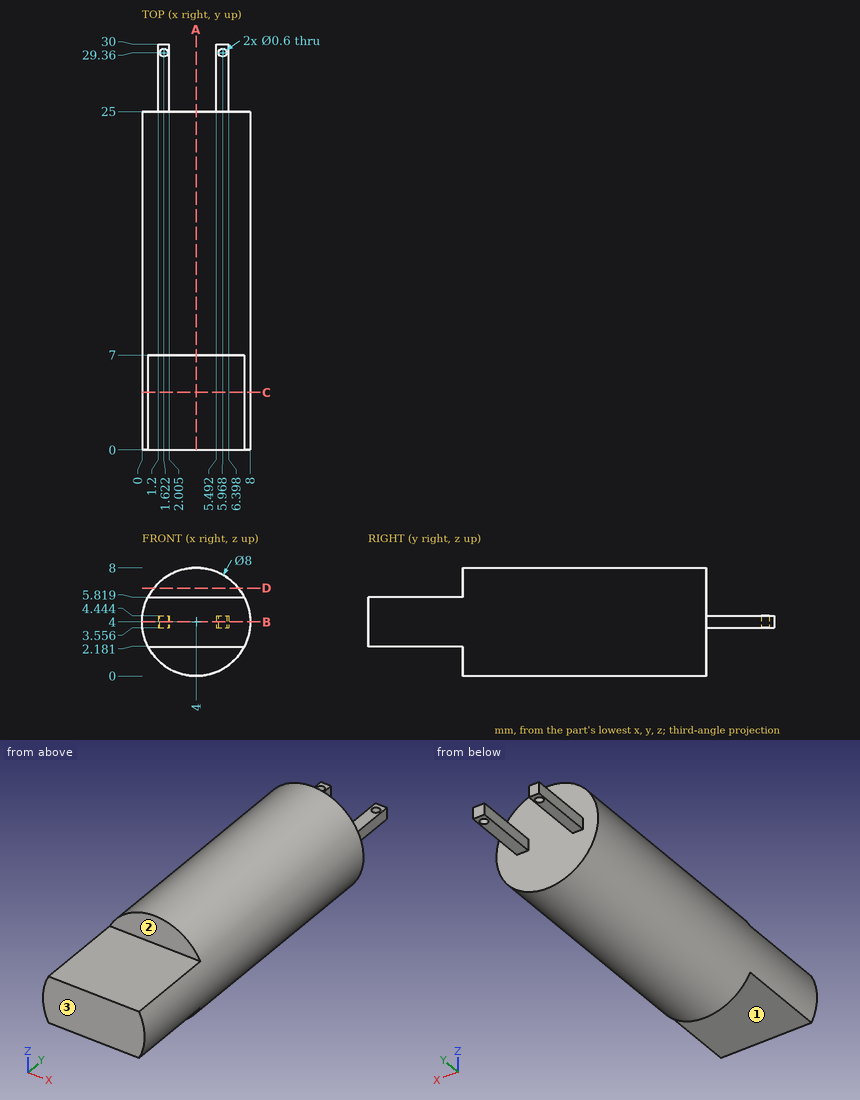
For this review, use the dimensioned drawing (mm, ordinates from the lowest corner) and the shaded views. A direction names the side the tool comes from. Give positions to 0.01 mm unless a question says otherwise; leave off trailing zeros. Loops run counter-clockwise (first coordinate to the right, second up) from the corner with the lowest first, then second, coordinate; pieces in that order, holes last. Notation, with made-up numbers: (5.25, 14.5) - (55.25, 14.5) arc R22 ccw to (55.25, 26.5) - close; hole circle Ø7 at (17, 86.25). An arc over 180 degrees is marked (long way). Write each question's results on one line, items separated by ' | '.
(1) For pin 1 Ø1.5 at (y, z) = (12.5, 2) entering from +X; pin 2 Ø1 at (x, y) = (6, 27.5) entering from -Z; pin 3 Ø0.9 at (x, y) = (2, 27) entering from +Z, all flat-tipped, find the tip position at first contact; note any pin that passes through.
Conclusion:
pin 1: x = 7.8 | pin 2: z = 3.56 | pin 3: z = 4.44
(2) For the marked faces 1, 2 and 3, list the 3-axis set-ups (+Z, -Z, +X, -X, +Y, -Y) from which the entire face can be reached by the end or side of a thin tool; tool diameter is ignored.
Conclusion:
face 1: -Z, +X, -X, -Y | face 2: +Z, +X, -X, -Y | face 3: +Z, -Z, +X, -X, -Y
(3) Take a section at D-D (z = 6.5). Give the boundary of the cut face in (x, y), then the cut area to 3 significant figures.
Conclusion:
outline: (0.88, 7) - (7.12, 7) - (7.12, 25) - (0.88, 25) - close | area: 112 mm^2
(4) Take a section at A-A (x = 4). Give the boundary of the cut face in (y, z).
Conclusion:
outline: (0, 2.18) - (7, 2.18) - (7, 0) - (25, 0) - (25, 8) - (7, 8) - (7, 5.82) - (0, 5.82) - close
(5) Take a section at B-B (z = 4). Give the boundary of the cut face in (x, y) (1 decimal).
Conclusion:
outline: (0, 0) - (8, 0) - (8, 25) - (6.4, 25) - (6.4, 30) - (5.5, 30) - (5.5, 25) - (2, 25) - (2, 30) - (1.2, 30) - (1.2, 25) - (0, 25) - close; hole circle Ø0.6 at (1.6, 29.4); hole circle Ø0.6 at (6, 29.4)
(6) For line 1 along X through (y, z) = (27.25, 4) (1 decimal); line 2 along Y through (x, z) = (3, 6.75); line 3 along Y through (x, z) = (3, 5.75), list the stretches that pass through material, from the lowest coordinate up.
Conclusion:
line 1: 1.2 to 2, 5.5 to 6.4 | line 2: 7 to 25 | line 3: 0 to 25
(7) Take a section at C-C (y = 4.25). Give the boundary of the cut face in (x, z).
Conclusion:
outline: (0.44, 2.18) - (7.56, 2.18) arc R4 ccw to (7.56, 5.82) - (0.44, 5.82) arc R4 ccw to start
